Can you work these out from the model? Positions are in its coordinate system, mm. Face numbers are marked on the shaded views. A direction names the side the tool comes from. Coordinates: 2 decimals unless noted, no trailing zeros. Loops run counter-clockwise (first coordinate to the right, second up) from the corner with the lowest first, then second, coordinate; pieces in that order, holes last. Notation, with made-up numbers: (-27.75, 85) -> (20.25, 85) arc R22 ccw to (20.25, 98) -> close; hole circle Ø2 at (0, 85). An arc over 180 degrees is marked (long way). Put each result on its own line as item: value. Start each with the question number.
Item 1: If we section it at A-A on x = 57: Please give me the cut outline in (y, z).
Item 2: If we section it at B-B on y = -15: Please give me the cut outline in (x, z).
Item 3: For the marked faces 3, 4 and 5, which set-ups out of +Z, -Z, +X, -X, +Y, -Y let a thin tool reach every point of the face, with its end or its side?
Item 4: We'd pull the mould along X, two halves only. Please class the marked faces 1 and 2: pulls with the +X half, pulls with the -X half, needs draft (parallel to the pull), parting line crosses it, or undercut.
Item 5: Please list where these lines run through material, in increasing order: L1, parallel to Z at x = 54, y = 0; L2, parallel to Z at x = 243, y = -11.5; L3, parallel to Y at x = 182, z = 25. Write a range as from..to.
Item 6: Will these pins go through, and if not, where does the flat tip stop? P1, Ø12.5, axis at x = 219, y = 4, coming from the -Z side; P2, Ø11.5, axis at x = 196.5, z = 20, coming from the -Y side; P3, Ø1.5, axis at y = 2, z = 12, coming from the +X side; P4, Ø1.5, axis at x = 62.5, z = 2.5, coming from the +Y side.
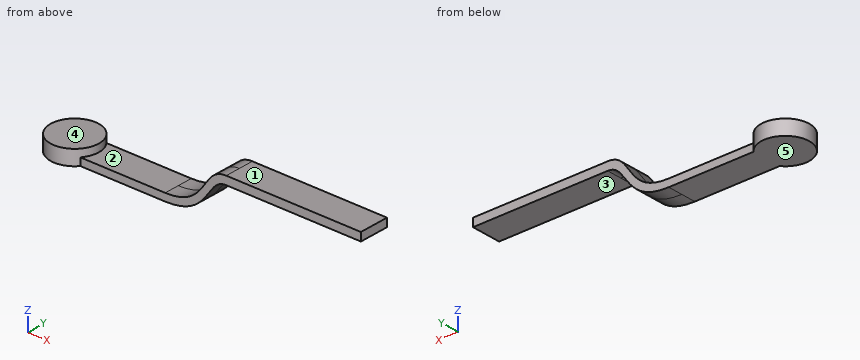
```python
from build123d import *

# Parameters (mm, degrees)
F0_W     = 87.8377447401
F0_H     = 6.35
F0_W_2   = 114.3
F0_H_2   = 6.9760140031
F1_DEPTH = 12.7


with BuildPart() as f1:
    # F0 (on Front) → F1 (new body, symmetric)
    with BuildSketch(Plane.XZ):
        with Locations((54.0722241176, -3.175)):
            Rectangle(F0_W, F0_H)
        with BuildLine():
            add(Edge.make_bspline(
                [(97.9910964877, 0), (135.2877169847, 0), (127.9766007824, 31.2006380408), (149.8604118824, 31.2006380408)],
                knots=[0, 0, 0, 0, 60.5302048045, 60.5302048045, 60.5302048045, 60.5302048045], degree=3))
            Line((97.9910964877, 0), (97.9910964877, -6.35))
            add(Edge.make_bspline(
                [(97.9910964877, -6.35), (136.9185000658, -6.35), (132.026180625, 24.2246240377), (149.8604118824, 24.2246240377)],
                knots=[0, 0, 0, 0, 60.2099120957, 60.2099120957, 60.2099120957, 60.2099120957], degree=3))
            Line((149.8604118824, 24.2246240377), (149.8604118824, 31.2006380408))
        make_face()
        with Locations((207.0104118824, 27.7126310393)):
            Rectangle(F0_W_2, F0_H_2)
    extrude(amount=F1_DEPTH, both=True)

    # F0 (on Front) → F2 (revolve)
    with BuildSketch(Plane.XZ):
        Polygon((10.1533517476, 6.35), (-10.1533517476, 6.35), (-10.1533517476, -6.35), (10.1533517476, -6.35), (10.1533517476, 0), align=None)
    revolve(axis=Axis((10.1533517476, 0, 0), (0, 0, -1)))


solid = f1.part
```
Solutions:
1. outline: (-12.7, -6.35) -> (12.7, -6.35) -> (12.7, 0) -> (-12.7, 0) -> close
2. outline: (-3.53, -6.35) -> (23.84, -6.35) -> (23.84, 6.35) -> (-3.53, 6.35) -> close
3. face 3: -Z, +X, +Y, -Y
3. face 4: +Z, -X, +Y, -Y
3. face 5: -Z, +X, -X, +Y, -Y
4. face 1: needs draft
4. face 2: undercut
5. L1: -6.35..0
5. L2: 24.22..31.2
5. L3: -12.7..12.7
6. P1: z = 24.22
6. P2: y = -12.7
6. P3: x = 134.61
6. P4: through
